```python
from build123d import *

# Parameters (mm, degrees)
F1_W           = 19.5961911231
F1_H           = 51.2615609914
F2_DEPTH       = 5
F3_R           = 1.35
F3_R_2         = 1.9
F4_DEPTH       = 4
F4_TAPER       = 5
F5_D           = 3
F5_DEPTH       = 25
F5_TIP         = 0.9012909285
F6_D           = 3.3
F6_DEPTH       = 25
F6_TIP         = 0.9914200214
F8_D           = 5.5
F8_DEPTH       = 25
F8_CBORE_D     = 9.75
F8_CBORE_DEPTH = 2
F8_TIP         = 1.6523667023


# Not quite as in the source:
# - a feature names something its author has since deleted; it is built from what else it names


with BuildPart() as f2:
    # F1 (on Top) → F2 (new body)
    with BuildSketch(Plane.XY):
        with Locations((0.1254314557, 10.8716255054)):
            Rectangle(F1_W, F1_H)
    extrude(amount=-F2_DEPTH)

    # F3 (on face) → F4 (join)
    with BuildSketch(Plane.XY):
        with Locations((-6, 32)):
            Circle(F3_R)
        with Locations((6, 32)):
            Circle(F3_R)
        with Locations((6, 12)):
            Circle(F3_R_2)
        with Locations((-6, 12)):
            Circle(F3_R_2)
        with Locations((6, -12)):
            Circle(F3_R)
        with Locations((-6, -12)):
            Circle(F3_R)
    extrude(amount=F4_DEPTH, taper=F4_TAPER)

    # F5 (one way)
    with BuildSketch(Plane(origin=(0, 0, 0), x_dir=(1, 0, 0), z_dir=(0, 0, -1))):
        with Locations((-6, -12), (6, -12)):
            Circle(F5_D / 2)
    extrude(amount=-F5_DEPTH, mode=Mode.SUBTRACT)
    with Locations(Plane(origin=(0, 0, 0), x_dir=(1, 0, 0), z_dir=(0, 0, -1))):
        with Locations((-6, -12), (6, -12)):
            with Locations((0, 0, -(F5_DEPTH + F5_TIP / 2))):  # 118° drill point
                Cone(0, F5_D / 2, F5_TIP, mode=Mode.SUBTRACT)

    # F6 (one way)
    with BuildSketch(Plane.XY):
        with Locations((6, 12), (-6, 12)):
            Circle(F6_D / 2)
    extrude(amount=-F6_DEPTH, mode=Mode.SUBTRACT)
    with Locations(Plane.XY):
        with Locations((6, 12), (-6, 12)):
            with Locations((0, 0, -(F6_DEPTH + F6_TIP / 2))):  # 118° drill point
                Cone(0, F6_D / 2, F6_TIP, mode=Mode.SUBTRACT)

    # F8
    with Locations(Plane.XY):
        with Locations((0, 0), (0, 25)):
            CounterBoreHole(F8_D / 2, F8_CBORE_D / 2, F8_CBORE_DEPTH, depth=F8_DEPTH)
            with Locations((0, 0, -(F8_DEPTH + F8_TIP / 2))):  # 118° drill point
                Cone(0, F8_D / 2, F8_TIP, mode=Mode.SUBTRACT)


solid = f2.part
```
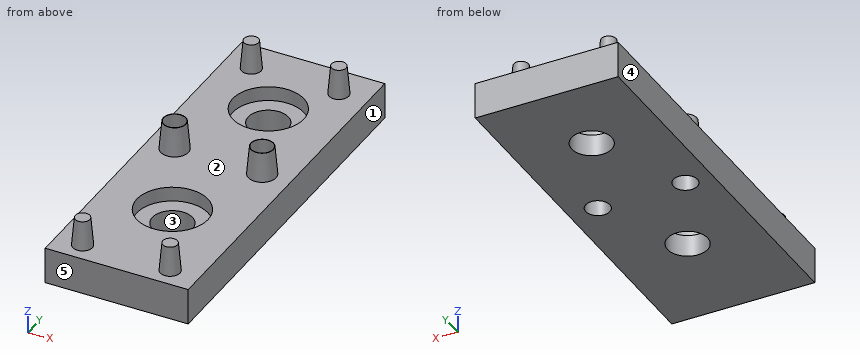
The listing builds one solid part. Answer for the finished solid, in the listing's coordinates (mm). Face numbers are marked on the shaded views. A direction names the side the tool comes from. Give positions to 0.01 mm unless a question says otherwise; leave off trailing zeros. Order: outer loops, then holes, each group sorted by start corner. A loop starts at its lowest first (then second) coordinate and runs counter-clockwise, first axis right, second up. Notation, with made-up numbers: (-3, -23) -> (49, -23) arc R33 ccw to (49, 5) -> close; hole circle Ø8 at (80, 48). An arc over 180 degrees is marked (long way). Answer as a JSON object with one key per item and string values. Group by question number.
Item 1: A tool of negligible diameter and unlimited length cuts with its end or side. For the marked faces 1 and 2, from which of +Z, -Z, +X, -X, +Y, -Y can it reach the whole face along a straight path? Write none if from no direction.
Item 2: The part is cut by section B-B on x = 0. Write down the section's boundary in (y, z) (3 decimals).
Item 3: Consider L1, parallel to Y at x = 0, z = -1 (3 decimals); L2, parallel to Y at x = 0, z = -3.15; L3, parallel to Y at x = 6, z = -1.7. Determine where each line is inside the solid, lowest interval first. Write a range as from..to.
Item 4: The part is cut by section C-C on z = -2.5. Write down the section's boundary in (x, y).
Item 5: Determine the mould class of the marked faces 3, 4 and 5 for opening direction X: pulls with the +X half, pulls with the -X half, needs draft (parallel to the pull), parting line crosses it, or undercut.
Item 6: Flat-ended cylindrical pins translate along their axes: pin 1 (10 mm diameter, centred on x = -1, y = 18.5, fed in from +Z); pin 2 (9 mm diameter, centred on x = 0, y = 0, fed in from -Z); pin 3 (3 mm diameter, centred on x = -1, y = 1.5, fed in from +Z). Find the tip coordinate at first contact, or state that the pin passes through.
Item 7: The part is cut by section A-A on y = 12. Write down the section's boundary in (x, z).
Item 8: The part is cut by section D-D on y = 0. Write down the section's boundary in (x, z) (3 decimals).
Result set:
{
 "1": {"face 1": "+Z, -Z, +X, +Y, -Y", "face 2": "+Z"},
 "2": {"outline": "(-14.759, -5) -> (-2.75, -5) -> (-2.75, -2) -> (-4.875, -2) -> (-4.875, 0) -> (-14.759, 0) -> close; (2.75, -5) -> (22.25, -5) -> (22.25, -2) -> (20.125, -2) -> (20.125, 0) -> (4.875, 0) -> (4.875, -2) -> (2.75, -2) -> close; (27.75, -5) -> (36.502, -5) -> (36.502, 0) -> (29.875, 0) -> (29.875, -2) -> (27.75, -2) -> close"},
 "3": {"L1": "-14.759..-4.875, 4.875..20.125, 29.875..36.502", "L2": "-14.76..-2.75, 2.75..22.25, 27.75..36.5", "L3": "-14.76..10.35, 13.65..36.5"},
 "4": {"outline": "(-9.67, -14.76) -> (9.92, -14.76) -> (9.92, 36.5) -> (-9.67, 36.5) -> close; hole circle Ø3.3 at (-6, 12); hole circle Ø5.5 at (0, 0); hole circle Ø5.5 at (0, 25); hole circle Ø3.3 at (6, 12)"},
 "5": {"face 3": "undercut", "face 4": "pulls with the -X half", "face 5": "needs draft"},
 "6": {"pin 1": "z = 0", "pin 2": "z = -5", "pin 3": "z = -2"},
 "7": {"outline": "(-9.67, -5) -> (-7.65, -5) -> (-7.65, 0) -> (-7.5, 0) -> (-7.5, 4) -> (-7.55, 4) -> (-7.9, 0) -> (-9.67, 0) -> close; (-4.5, 0) -> (-4.35, 0) -> (-4.35, -5) -> (4.35, -5) -> (4.35, 0) -> (4.5, 0) -> (4.5, 4) -> (4.45, 4) -> (4.1, 0) -> (-4.1, 0) -> (-4.45, 4) -> (-4.5, 4) -> close; (7.5, 0) -> (7.65, 0) -> (7.65, -5) -> (9.92, -5) -> (9.92, 0) -> (7.9, 0) -> (7.55, 4) -> (7.5, 4) -> close"},
 "8": {"outline": "(-9.673, -5) -> (-2.75, -5) -> (-2.75, -2) -> (-4.875, -2) -> (-4.875, 0) -> (-9.673, 0) -> close; (2.75, -5) -> (9.924, -5) -> (9.924, 0) -> (4.875, 0) -> (4.875, -2) -> (2.75, -2) -> close"}
}
